For this review, take the finished solid that the model builds, in its own axes (mm). Coordinates: 2 decimals unless noted, no trailing zeros. Loops run counter-clockwise (first coordinate to the right, second up) from the corner with the lowest first, then second, coordinate; pieces in that order, holes last. Notation, with made-up numbers: M 41.5,15 L 45.5,15 A33 ccw 45.5,43 Z; hole C -17,72.25 d4. An arc over 180 degrees is marked long. Write item = value, one per line.
from build123d import *

# Parameters (mm, degrees)
F0_R     = 25.4
F0_R_2   = 23.7717418162
F1_DEPTH = 25.4
F2_R     = 25.4
F2_R_2   = 23.7717418162
F3_DEPTH = 3
F4_R     = 7.62


# Not quite as in the source:
# - a fillet or chamfer that OpenCascade refuses, or shapes differently, is made with other operations: its cross-section is extruded or revolved along the edge and cut away or added


with BuildPart() as f1:
    # F0 (on Top) → F1 (new body)
    with BuildSketch(Plane.XY):
        Circle(F0_R)
        Circle(F0_R_2, mode=Mode.SUBTRACT)
    extrude(amount=F1_DEPTH)

    # F2 (on face) → F3 (join)
    with BuildSketch(Plane.XY.offset(25.4)):
        Circle(F2_R)
        Circle(F2_R_2, mode=Mode.SUBTRACT)
        Circle(F2_R)
    extrude(amount=F3_DEPTH)

    # F4
    f4_edges = [f1.edges().sort_by_distance(p)[0] for p in [
        (-25.4, 0, 28.4),
    ]]
    fillet(f4_edges, radius=F4_R)

    # F5: fillet of radius 5.08 on 1 edges, made by hand

    # F5_s1 → F5_t2 (revolve, cut)
    with BuildSketch(Plane.XZ):
        with BuildLine():
            ThreePointArc((25.4, 0), (24.1965700457, 1.6935203443), (23.7717418162, 3.7271810305))
            Line((23.7717418162, 3.7271810305), (23.7717418162, 0))
            Line((23.7717418162, 0), (25.4, 0))
        make_face()
    revolve(axis=Axis((0, 0, 0), (0, 0, 1)), mode=Mode.SUBTRACT)


solid = f1.part
Q1. Draft analysis for pull direction X (two halves, no side actions). For faces 1 (the face through (-5.153, -23.206, 14.412)), 2 (the face through (-5.506, -24.796, 10.245)), 3 (the face through (0, 0, 28.4)), state which applies: +X half, -X half, draft (parallel to the pull), parting line (faces both ways), or undercut.
Solved:
face_1 = undercut
face_2 = parting line
face_3 = draft
Q2. Add section A-A (y = 0). Write out the cut boundary in (x, z), and give its area (3 significant figures).
Solved:
outline = M -25.4,0 A5.08 ccw -23.77,3.73 L -23.77,25.4 L 23.77,25.4 L 23.77,3.73 A5.08 ccw 25.4,0 L 25.4,20.78 A7.62 ccw 17.78,28.4 L -17.78,28.4 A7.62 ccw -25.4,20.78 Z
area = 206 mm²
Q3. Add section C-C (z = 8.5). Write out the cut boundary in (x, y), and give its area (3 significant figures).
Solved:
outline = C 0,0 d50.8; hole C 0,0 d47.54
area = 252 mm²
Q4. For pin 1 Ø2 at (x, z) = (4, 16.5) entering from -Y; pin 2 Ø5 at (y, z) = (-14.5, 23.5) entering from -X; pin 3 Ø1 at (y, z) = (7.5, 4.5) entering from +X, all flat-tipped, find the tip position at first contact; note any pin that passes through.
Solved:
pin_1 = -25.22
pin_2 = -22.05
pin_3 = 24.42
Q5. For line 1 along Y through (x, z) = (0, 16.75); line 2 along X through (y, z) = (15.5, 24.5); line 3 along Z through (x, y) = (15.5, -7.5), list the stretches that pass through material, from the lowest coordinate up.
Solved:
line_1 = -25.4 to -23.77, 23.77 to 25.4
line_2 = -18.88 to -18.02, 18.02 to 18.88
line_3 = 25.4 to 28.4
Q6. Add section D-D (z = 21.75). Write out the cut boundary in (x, y).
Solved:
outline = C 0,0 d50.68; hole C 0,0 d47.54
